from build123d import *

# Parameters (mm, degrees)
F0_W     = 100
F0_H     = 100
F1_DEPTH = 25
F2_SIZE  = 24.99999


# Not quite as in the source:
# - a fillet or chamfer is up to 0.001 mm smaller than in the source, because OpenCascade refuses the exact size


with BuildPart() as f1:
    # F0 (on Front) → F1 (new body)
    with BuildSketch(Plane.XZ):
        Rectangle(F0_W, F0_H)
    extrude(amount=-F1_DEPTH)

    # F2 (size 25 in the source; OpenCascade refuses exactly that, so slightly less here)
    f2_edges = [f1.edges().sort_by_distance(p)[0] for p in [
        (50, 25, 0),
        (-50, 25, 0),
    ]]
    chamfer(f2_edges, length=F2_SIZE)


solid = f1.part
Work out the finished part from the listing and answer in its coordinate system (mm). Give positions to 0.01 mm unless a question says otherwise; leave off trailing zeros. Write each loop counter-clockwise with the first axis right and the second up, starting at its lowest first coordinate (ties: lowest second). Pieces come first, ordered by that corner, then holes. Notation, with made-up numbers: M 85.25,-25.75 L 141.25,-25.75 A28 cw 141.25,-7.75 Z; hole C -23.75,-39.75 d5. An arc over 180 degrees is marked long. Answer as CSV lines item,"result".
Q1. A cutting plane is placed at C-C on x = -26.5. Write down the section's boundary in (y, z), plus the area to 3 significant figures.
A:
outline,"M 0,-50 L 23.5,-50 L 23.5,50 L 0,50 Z"
area,"2,350 mm²"
Q2. Given P1, Ø2, axis at y = 9, z = 33.5, coming from the -X side; P2, Ø5, axis at y = 20.5, z = -24.5, coming from the -X side; P3, Ø10, axis at y = 18, z = -20.5, coming from the +X side, each flat-ended and moving along its own axis, determine where each tip first touches the part or whether it passes through.
A:
P1,"stops at x = -42"
P2,"stops at x = -32"
P3,"stops at x = 37"
Q3. Find the intervals of material crossed by probe 1 along X at (y, z) = (14.25, -27.5); probe 2 along X at (y, z) = (18.25, -34); probe 3 along Y at (x, z) = (-31.5, 40.5), in increasing order. Write a range as [from, to].
A:
probe 1,"x = [-35.75, 35.75]"
probe 2,"x = [-31.75, 31.75]"
probe 3,"y = [0, 18.5]"
